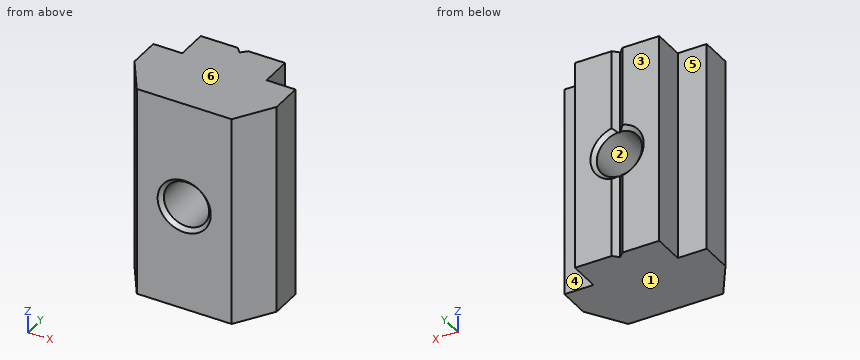
```python
from build123d import *

# Parameters (mm, degrees)
EXTRUDE_1_DEPTH     = 10
SKETCH_2_R          = 2.15
CUT_EXTRUDE_1_DEPTH = 16.356187678
CUT_EXTRUDE_2_DEPTH = 10
CHAMFER_1_SIZE      = 0.375


with BuildPart() as part:
    # 草图1 → 凸台-拉伸1 (new, symmetric)
    with BuildSketch(Plane.XY):
        Polygon((-4.5, 0), (4.5, 0), (6.75, 3.464696169), (6.75, 6.5), (4, 6.5), (4, 9.5), (-4, 9.5), (-4, 6.5), (-6.75, 6.5), (-6.75, 3.464696169), align=None)
    extrude(amount=EXTRUDE_1_DEPTH, both=True)

    # 草图2 → 切除-拉伸1 (cut, through all)
    with BuildSketch(Plane(origin=(0, 9.5, 0), x_dir=(1, 0, 0), z_dir=(0, 1, 0))):
        with Locations(Location((0, 0, 0), (0, 0, 180))):
            Circle(SKETCH_2_R)
    extrude(amount=-CUT_EXTRUDE_1_DEPTH, mode=Mode.SUBTRACT)

    # 草图3 → 切除-拉伸2 (cut, symmetric)
    with BuildSketch(Plane.XY):
        Polygon((-0.509116882, 9.5), (0, 8.990883118), (0.509116882, 9.5), (0, 10.009116882), align=None)
    extrude(amount=CUT_EXTRUDE_2_DEPTH, both=True, mode=Mode.SUBTRACT)

    # 倒角1
    chamfer_1_edges = [part.edges().sort_by_distance(p)[0] for p in [
        (2.15, 0, 0),
        (2.15, 9.5, 0),
        (-1.690724889, 9.5, -1.32813755),
    ]]
    chamfer(chamfer_1_edges, length=CHAMFER_1_SIZE)


solid = part.part
```
Geometry check sheet. Reference: the model listing, model coordinates, mm. Face numbers are marked on the shaded views. A direction names the side the tool comes from. Coordinates: 2 decimals unless noted, no trailing zeros. Write each loop counter-clockwise with the first axis right and the second up, starting at its lowest first coordinate (ties: lowest second). Pieces come first, ordered by that corner, then holes. Notation, with made-up numbers: M 59,-19 L 94,-19 A13 ccw 94,0 Z; hole C 66.25,13.5 d1. An arc over 180 degrees is marked long. Use one line per item in the form item = value. Start each with the question number.
1) Go/stop test with flat-tipped pins: pin 1 Ø2 at (x, z) = (-5.5, -3) entering from +Y; pin 2 Ø1.5 at (y, z) = (2, 2.5) entering from +X; pin 3 Ø1.5 at (y, z) = (8, -3.5) entering from -X. Record where each tip stops, or that it passes through.
2) Section check A-A on z = 0. Enter the section's corners in (x, y) (3 decimals).
3) Section check B-B on y = 5.25. Enter the section's corners in (x, z), and give its area (3 significant figures).
4) Section check D-D on y = 8.25. Enter the section's corners in (x, z).
5) Set-up check for the marked faces 4, 5 and 6: record each of +Z, -Z, +X, -X, +Y, -Y from which the full face is reachable in a straight line by a thin tool's end or side.
6) Section check C-C on z = 8.25. Enter the section's corners in (x, y).
7) Release check for a two-part mould opening along Z. For the marked faces 1, 2 and 3 record: pulls with the +Z half, pulls with the -Z half, needs draft (parallel to the pull), parting line crosses it, or undercut.
8) Thickness scan on probe 1 along Z at (x, y) = (0, 4); probe 2 along X at (y, z) = (7, 0); probe 3 along X at (y, z) = (5, 0). Record the ranges inside material, lowest first. Write a range as from..to.
Responses:
q1.pin_1 = 6.5
q1.pin_2 = 6.29
q1.pin_3 = -4
q2.outline = M -6.75,3.465 L -4.5,0 L -2.525,0 L -2.15,0.375 L -2.15,9.125 L -2.525,9.5 L -4,9.5 L -4,6.5 L -6.75,6.5 Z; M 2.15,0.375 L 2.525,0 L 4.5,0 L 6.75,3.465 L 6.75,6.5 L 4,6.5 L 4,9.5 L 2.525,9.5 L 2.15,9.125 Z
q3.outline = M -6.75,-10 L 6.75,-10 L 6.75,10 L -6.75,10 Z; hole C 0,0 d4.3
q3.area = 255 mm2
q4.outline = M -4,-10 L 4,-10 L 4,10 L -4,10 Z; hole C 0,0 d4.3
q5.face_4 = +Z, -Z, +X, +Y
q5.face_5 = +Z, -Z, -X, +Y
q5.face_6 = +Z, +X, -X, +Y, -Y
q6.outline = M -6.75,3.46 L -4.5,0 L 4.5,0 L 6.75,3.46 L 6.75,6.5 L 4,6.5 L 4,9.5 L 0.51,9.5 L 0,8.99 L -0.51,9.5 L -4,9.5 L -4,6.5 L -6.75,6.5 Z
q7.face_1 = pulls with the -Z half
q7.face_2 = undercut
q7.face_3 = needs draft
q8.probe_1 = -10..-2.15, 2.15..10
q8.probe_2 = -4..-2.15, 2.15..4
q8.probe_3 = -6.75..-2.15, 2.15..6.75
